CAD build for the part. Positions are in the model's coordinates, mm. Face numbers are marked on the shaded views. A direction names the side the tool comes from. Give positions to 0.01 mm unless a question says otherwise; leave off trailing zeros. Loops run counter-clockwise (first coordinate to the right, second up) from the corner with the lowest first, then second, coordinate; pieces in that order, holes last.
Item 1: Which spindle directions (+Z, -Z, +X, -X, +Y, -Y) get a long thin tool onto all of the face, cutting with end or side? Do the marked faces 1, 2 and 3. Say none if no direction does.
Item 2: Probe probe 1 along Z at (x, y) = (10, -1.5) (3 decimals); probe 2 along X at (y, z) = (-1.25, 1.5); probe 3 along Y at (x, z) = (-10.75, 6). List the from-to ranges inside material, lowest first.
Item 3: Saw through at A-A on x = -10. Give the cut face in (y, z) (3 decimals), plus the area to 3 significant figures.
Item 4: Saw through at B-B on x = 0. Give the cut face in (y, z), plus the area to 3 significant figures.
Item 5: Mould opens along Y. For the marked faces 4, 5 and 6 say: released by +Y, released by -Y, zero draft, split by the parting line, or undercut.
Item 6: Saw through at D-D on x = 11.5. Give the cut face in (y, z) (3 decimals), plus the area to 3 significant figures.
Item 7: Drop flat-ended pins along their axis: P1, Ø6, axis at x = 10, z = 0.23, coming from the -Y side; P2, Ø1.5, axis at x = 3.5, z = -1, coming from the -Y side; P3, Ø4, axis at y = -11.5, z = -2, coming from the -X side. Give the stop position or say it passes through.
Item 8: Saw through at C-C on y = -7. Give the cut face in (x, z), plus the area to 3 significant figures.
from build123d import *

# Parameters (mm, degrees)
SKETCH_1_W          = 29
SKETCH_1_H          = 13
EXTRUDE_1_DEPTH     = 2
SKETCH_2_R          = 2.5
CUT_EXTRUDE_1_DEPTH = 17.015617378
SKETCH_3_R          = 6
EXTRUDE_2_DEPTH     = 5


with BuildPart() as part:
    # Sketch 1 → Extrude 1 (new body)
    with BuildSketch(Plane(origin=(0, 0, 0), x_dir=(1, 0, 0), z_dir=(0, 1, 0))):
        Rectangle(SKETCH_1_W, SKETCH_1_H)
    extrude(amount=-EXTRUDE_1_DEPTH)

    # Sketch 2 → Cut-Extrude 1 (cut, through all)
    with BuildSketch(Plane(origin=(0, 0, 0), x_dir=(1, 0, 0), z_dir=(0, 1, 0))):
        with Locations(Location((-10, -0.234995389, 0), (0, 0, 270))):
            Circle(SKETCH_2_R)
        with Locations(Location((10, -0.234995389, 0), (0, 0, 90))):
            Circle(SKETCH_2_R)
    extrude(amount=-CUT_EXTRUDE_1_DEPTH, mode=Mode.SUBTRACT)

    # Sketch 3 → Extrude 2 (add, symmetric)
    with BuildSketch(Plane.XY):
        with Locations((0, -7)):
            Circle(SKETCH_3_R)
    extrude(amount=EXTRUDE_2_DEPTH, both=True)


solid = part.part
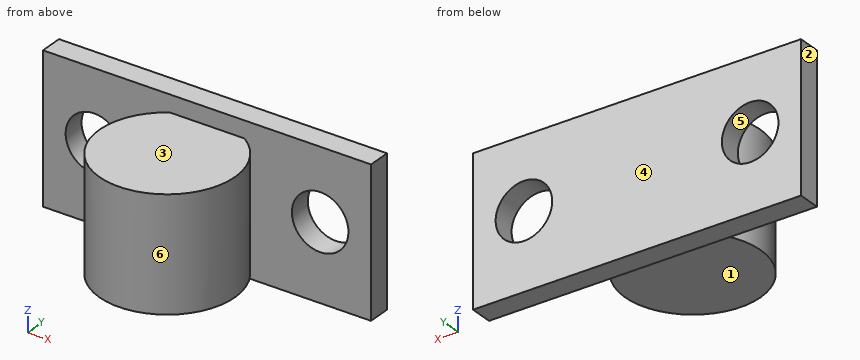
Results below:
1. face 1: -Z, +X, -X, -Y
1. face 2: +Z, -Z, -X, +Y, -Y
1. face 3: +Z, +X, -X, -Y
2. probe 1: z = -6.5 to -2.265, 2.735 to 6.5
2. probe 2: x = -14.5 to -12.16, -7.84 to 7.84, 12.16 to 14.5
2. probe 3: y = -2 to 0
3. outline: (-2, -6.5) - (0, -6.5) - (0, -2.265) - (-2, -2.265) - close; (-2, 2.735) - (0, 2.735) - (0, 6.5) - (-2, 6.5) - close
3. area: 16.0 mm2
4. outline: (-13, -5) - (-2, -5) - (-2, -6.5) - (0, -6.5) - (0, 6.5) - (-2, 6.5) - (-2, 5) - (-13, 5) - close
4. area: 136 mm2
5. face 4: released by +Y
5. face 5: zero draft
5. face 6: undercut
6. outline: (-2, -6.5) - (0, -6.5) - (0, -1.765) - (-2, -1.765) - close; (-2, 2.235) - (0, 2.235) - (0, 6.5) - (-2, 6.5) - close
6. area: 18.0 mm2
7. P1: stops at y = -2
7. P2: stops at y = -12.33
7. P3: stops at x = -5.45
8. outline: (-6, -5) - (6, -5) - (6, 5) - (-6, 5) - close
8. area: 120 mm2
